from build123d import *

# Parameters (mm, degrees)
SKETCH1_R           = 3.175
SKETCH1_R_2         = 1.397
BOSS_EXTRUDE1_DEPTH = 3.175


with BuildPart() as part:
    # Sketch1 → Boss-Extrude1 (new body)
    with BuildSketch(Plane.XY):
        with BuildLine():
            Line((0, 58.42), (0, 53.213))
            Line((0, 53.213), (3.048, 53.213))
            Line((3.048, 53.213), (3.048, 6.35))
            Line((3.048, 6.35), (0, 6.35))
            Line((0, 6.35), (0, 6.731))
            Line((0, 6.731), (-3.556, 6.731))
            ThreePointArc((-3.556, 6.731), (-1.31093597, 5.80106403), (-0.381, 3.556))
            ThreePointArc((-0.381, 3.556), (-3.556, 0.381), (-6.731, 3.556))
            Line((-6.731, 3.556), (-6.731, 0))
            Line((-6.731, 0), (-10.287, 0))
            Line((-10.287, 0), (-10.287, -3.048))
            Line((-10.287, -3.048), (-45.847, -3.048))
            Line((-45.847, -3.048), (-45.847, 0))
            Line((-45.847, 0), (-49.403, 0))
            Line((-49.403, 0), (-49.403, 3.556))
            ThreePointArc((-49.403, 3.556), (-54.82306403, 1.31093597), (-52.578, 6.731))
            Line((-52.578, 6.731), (-56.134, 6.731))
            Line((-56.134, 6.731), (-56.134, 6.35))
            Line((-56.134, 6.35), (-59.182, 6.35))
            Line((-59.182, 6.35), (-59.182, 53.213))
            Line((-59.182, 53.213), (-56.134, 53.213))
            Line((-56.134, 53.213), (-56.134, 58.42))
            Line((-56.134, 58.42), (-52.578, 58.42))
            ThreePointArc((-52.578, 58.42), (-55.753, 61.595), (-52.578, 64.77))
            Line((-52.578, 64.77), (-59.182, 64.77))
            ThreePointArc((-59.182, 64.77), (-60.978051224, 64.026051224), (-61.722, 62.23))
            Line((-61.722, 62.23), (-61.722, -3.048))
            ThreePointArc((-61.722, -3.048), (-60.978051224, -4.844051224), (-59.182, -5.588))
            Line((-59.182, -5.588), (3.048, -5.588))
            ThreePointArc((3.048, -5.588), (4.844051224, -4.844051224), (5.588, -3.048))
            Line((5.588, -3.048), (5.588, 62.23))
            ThreePointArc((5.588, 62.23), (4.844051224, 64.026051224), (3.048, 64.77))
            Line((3.048, 64.77), (-3.556000021, 64.77))
            ThreePointArc((-3.556000021, 64.77), (-1.310935977, 63.840064038), (-0.381, 61.595))
            ThreePointArc((-0.381, 61.595), (-1.31093597, 59.34993597), (-3.556, 58.42))
            Line((-3.556, 58.42), (0, 58.42))
        make_face()
        with Locations((-52.578, 61.595)):
            Circle(SKETCH1_R)
        with Locations((-52.578, 61.595)):
            Circle(SKETCH1_R_2, mode=Mode.SUBTRACT)
        with Locations((-3.556, 61.595)):
            Circle(SKETCH1_R)
        with Locations((-3.556, 61.595)):
            Circle(SKETCH1_R_2, mode=Mode.SUBTRACT)
        with Locations((-52.578, 3.556)):
            Circle(SKETCH1_R)
        with Locations((-52.578, 3.556)):
            Circle(SKETCH1_R_2, mode=Mode.SUBTRACT)
        with Locations((-3.556, 3.556)):
            Circle(SKETCH1_R)
        with Locations((-3.556, 3.556)):
            Circle(SKETCH1_R_2, mode=Mode.SUBTRACT)
    extrude(amount=BOSS_EXTRUDE1_DEPTH)


solid = part.part
Could you check a few things on this model? Use its own coordinates, in mm. A direction names the side the tool comes from. Round coordinates to 2 decimals unless told otherwise and drop trailing zeros. Order: outer loops, then holes, each group sorted by start corner. A loop starts at its lowest first (then second) coordinate and runs counter-clockwise, first axis right, second up. Notation, with made-up numbers: M 20,77.5 L 39,77.5 A20 cw 39,96.5 Z; hole C 2.5,-36 d7. An arc over 180 degrees is marked long. One line per item, written item: value.
(1) Imagine slicing it at A-A (y = 50). Write out the boundary of the cut face in (x, z) (3 decimals).
Ans:
outline: M -61.722,0 L -59.182,0 L -59.182,3.175 L -61.722,3.175 Z; M 3.048,0 L 5.588,0 L 5.588,3.175 L 3.048,3.175 Z
(2) Imagine slicing it at B-B (x = -43). Write out the boundary of the cut face in (y, z) (3 decimals).
Ans:
outline: M -5.588,0 L -3.048,0 L -3.048,3.175 L -5.588,3.175 Z
(3) If we mould it in two halves opening along X, with no side actions, what happens to faces 4 (the cylindrical face through (-61, -4.82, 1.57)), 5 (the cylindrical face through (-5.8, 5.8, 1.6)), 6 (the flat face through (-28, -4, 3.175))? For each: released by +X, released by -X, zero draft, split by the parting line, or undercut.
Ans:
face 4: released by -X
face 5: undercut
face 6: zero draft
(4) I'm going to push flat-ended pins straight in: P1, Ø4.5, axis at x = -3.556, y = 3.556, coming from the +Z side (3 decimals); P2, Ø1.7, axis at x = -3.556, y = 61.595, coming from the -Z side. Where does each tip first touch, or does it pass through?
Ans:
P1: stops at z = 3.175
P2: passes through
(5) Imagine slicing it at C-C (z = 2.05). Count the separate pieces of the cut face and the enclosed holes in it, and give its area (3 significant figures).
Ans:
separate pieces: 1
enclosed holes: 4
area: 839 mm^2
(6) I need wall thicknesses on line 1 along Y through (x, z) = (-3.5, 0.7); line 2 along X through (y, z) = (37, 0.8); line 3 along X through (y, z) = (1, 1.25). Which ranges of each line are inside material? Lowest first, please. Write a range as from..to.
Ans:
line 1: y = -5.59..2.16, 4.95..6.73, 58.42..60.2, 62.99..64.77
line 2: x = -61.72..-59.18, 3.05..5.59
line 3: x = -61.72..-49.4, -6.73..5.59
(7) Which directions (+Z, -Z, +X, -X, +Y, -Y) give clear straight access to the entire face, cutting with the end or side of a thin tool? Please do faces 1 (the flat face through (-45.847, -2, 2)), 2 (the flat face through (-56, 64.77, 2)), 3 (the cylindrical face through (-6.73, 61.66, 1.57)).
Ans:
face 1: +Z, -Z, +Y
face 2: +Z, -Z, +X, -X, +Y
face 3: +Z, -Z
